```python
from build123d import *

# Parameters (mm, degrees)
SKETCH1_R           = 2
SKETCH1_R_2         = 3.5
SKETCH1_W           = 9.000072
SKETCH1_H           = 2
SKETCH1_W_2         = 5
BOSS_EXTRUDE1_DEPTH = 4


with BuildPart() as part:
    # Sketch1 → Boss-Extrude1 (new body)
    with BuildSketch(Plane.XY):
        with BuildLine():
            Line((-12.978640908, -18), (-12.978640908, -24))
            Line((-12.978640908, -24), (23.021359092, -24))
            Line((23.021359092, -24), (23.021359092, -18))
            ThreePointArc((23.021359092, -18), (32.58126188, -15.140073441), (39, -7.5))
            ThreePointArc((39, -7.5), (45.227131985, 9.097629123), (47.343034567, 26.698237678))
            ThreePointArc((47.343034567, 26.698237678), (46.561018226, 46.955835458), (44.219623828, 67.092858318))
            Line((44.219623828, 67.092858318), (28.140376172, 69.067141682))
            Line((28.140376172, 69.067141682), (26.638766331, 75.523635508))
            Line((26.638766331, 75.523635508), (10.441233669, 75.806364492))
            Line((10.441233669, 75.806364492), (8.1, 82.51))
            Line((8.1, 82.51), (-8.1, 82.51))
            Line((-8.1, 82.51), (-14.491217975, 82.280462515))
            Line((-14.491217975, 82.280462515), (-30.688782025, 81.999537485))
            ThreePointArc((-30.688782025, 81.999537485), (-37.567707395, 47.245827753), (-37.052658257, 11.821617405))
            ThreePointArc((-37.052658257, 11.821617405), (-29.300451665, -6.548172019), (-12.978640908, -18))
        make_face()
        with Locations((38.147341743, 11.821617405)):
            Circle(SKETCH1_R, mode=Mode.SUBTRACT)
        with Locations((-24.678960076, 61.651218734)):
            Circle(SKETCH1_R_2, mode=Mode.SUBTRACT)
        with Locations((1.521420673, 61.651218734)):
            Circle(SKETCH1_R_2, mode=Mode.SUBTRACT)
        with Locations((14.86306514, 46.821617405)):
            Circle(SKETCH1_R_2, mode=Mode.SUBTRACT)
        with Locations((38.147341743, 46.821617405)):
            Circle(SKETCH1_R_2, mode=Mode.SUBTRACT)
        with Locations((-31.681501662, 43.456405989)):
            Circle(SKETCH1_R, mode=Mode.SUBTRACT)
        with Locations((-14, -9.124358763)):
            Circle(SKETCH1_R, mode=Mode.SUBTRACT)
        with Locations((0, 77.51)):
            Rectangle(SKETCH1_W, SKETCH1_H, mode=Mode.SUBTRACT)
        Polygon((-4, -2.5), (0, -2.5), (0, 0), (12, 0), (12, -2.5), (16, -2.5), (16, -12.5), (12, -12.5), (12, -15), (0, -15), (0, -12.5), (-4, -12.5), align=None, mode=Mode.SUBTRACT)
        with Locations((35.147341743, 56.321617405)):
            Rectangle(SKETCH1_W_2, SKETCH1_H, mode=Mode.SUBTRACT)
        Polygon((-27.019995137, 78.062566115), (-18.021276454, 78.218636824), (-17.986594351, 76.218937559), (-26.985313034, 76.062866849), align=None, mode=Mode.SUBTRACT)
        with Locations((17.86306514, 56.321617405)):
            Rectangle(SKETCH1_W_2, SKETCH1_H, mode=Mode.SUBTRACT)
        with Locations((-0.478579327, 71.151218734)):
            Rectangle(SKETCH1_W_2, SKETCH1_H, mode=Mode.SUBTRACT)
        Polygon((13.970839752, 71.744145677), (13.935934939, 69.744450286), (22.934636184, 69.587377372), (22.969540997, 71.587072762), align=None, mode=Mode.SUBTRACT)
        Polygon((40.15901604, 63.561398961), (31.226029212, 64.658231826), (30.982290526, 62.673139523), (39.915277354, 61.576306658), align=None, mode=Mode.SUBTRACT)
        Polygon((1.632632483, 35.912105076), (1.005748572, 29.944943559), (-18.884789816, 32.034556594), (-18.257905905, 38.00171811), align=None, mode=Mode.SUBTRACT)
        with Locations((-22.678960076, 71.151218734)):
            Rectangle(SKETCH1_W_2, SKETCH1_H, mode=Mode.SUBTRACT)
        Polygon((0.065422707, 20.994201285), (-1.188345114, 9.059878252), (-21.078883502, 11.149491286), (-19.825115681, 23.083814319), align=None, mode=Mode.SUBTRACT)
        Polygon((-9.666, 24.072796069), (-9.153, 28.955923243), (-23.205665371, 30.432234852), (-22.787742764, 34.410342529), (-30.743958119, 35.246187743), (-31.161880726, 31.268080066), (-34.143965433, 31.581364852), (-34.656965433, 26.698237678), (-31.674880726, 26.384952891), (-32.092803333, 22.406845214), (-24.136587978, 21.571), (-23.718665371, 25.549107678), align=None, mode=Mode.SUBTRACT)
    extrude(amount=BOSS_EXTRUDE1_DEPTH)


solid = part.part
```
CAD build for the part. Positions are in the model's coordinates, mm. A direction names the side the tool comes from. Round coordinates to 2 decimals unless told otherwise and drop trailing zeros. Order: outer loops, then holes, each group sorted by start corner. A loop starts at its lowest first (then second) coordinate and runs counter-clockwise, first axis right, second up. Notation, with made-up numbers: (28, 48.25) - (79, 48.25) arc R20 cw to (79, 55.25) - close; hole circle Ø2 at (9.25, 12). An arc over 180 degrees is marked (long way). Answer in a Markdown table with one row per item. Add a question column.
(1) Band-saw the part on B-B on z = 2.15. Count the separate pieces of the cut face and the enclosed holes in it, and give its area (3 significant figures).
(2) Probe L1, parallel to X at y = 59, z = 0.55 (3 decimals); L2, parallel to Y at x = 19, z = 0.5; L3, parallel to X at y = 70.5, z = 1.85. List the from-to ranges inside material, lowest first. Write a range as [from, to].
(3) 3-axis set-ups, long thin cutter, end or side, ignore diameter. For faces 4 (the face through (4, 30, 0)), 5 (the face through (0, -1, 2)): which of +Z, -Z, +X, -X, +Y, -Y reach the whole face in a straight line?
(4) Mould opens along X. For faces 1 (the face through (4, 30, 4)), 2 (the face through (-0.553, 15.111, 1.972)), 3 (the face through (27.4, 72.25, 1.97)) say: +X half, -X half, draft (parallel to the pull), parting line (faces both ways), or undercut.
(5) Band-saw the part on A-A on y = 1.5. List the corners of the cut face in (x, z), and give its area (3 significant figures).
(6) Drop flat-ended pins along their axis: pin 1 Ø2 at (y, z) = (-9, 1.5) entering from +X; pin 2 Ø0.6 at (y, z) = (70.5, 2) entering from -X; pin 3 Ø0.6 at (y, z) = (56, 2.5) entering from -X. Give the stop position or say it passes through.
Data:
| question | item | result |
|---|---|---|
| 1 | separate pieces | 1 |
| 1 | enclosed holes | 19 |
| 1 | area | 6,630 mm^2 |
| 2 | L1 | x = [-36.085, -26.964], [-22.394, -0.764], [3.806, 45.35] |
| 2 | L2 | y = [-24, 55.32], [57.32, 69.66], [71.66, 75.66] |
| 2 | L3 | x = [-33.81, -25.18], [-20.18, -2.98], [2.02, 13.95], [22.95, 27.81] |
| 3 | face 4 | -Z, +X, -X, +Y, -Y |
| 3 | face 5 | +Z, -Z |
| 4 | face 1 | draft |
| 4 | face 2 | undercut |
| 4 | face 3 | +X half |
| 5 | outline | (-34.21, 0) - (42.94, 0) - (42.94, 4) - (-34.21, 4) - close |
| 5 | area | 309 mm^2 |
| 6 | pin 1 | stops at x = 38.77 |
| 6 | pin 2 | stops at x = -33.88 |
| 6 | pin 3 | stops at x = -36.59 |
